Source: CAD feature listing. Evaluate the final solid. Frame: model axes, mm. Give positions to 0.01 mm unless a question says otherwise; leave off trailing zeros. Loops run counter-clockwise (first coordinate to the right, second up) from the corner with the lowest first, then second, coordinate; pieces in that order, holes last.
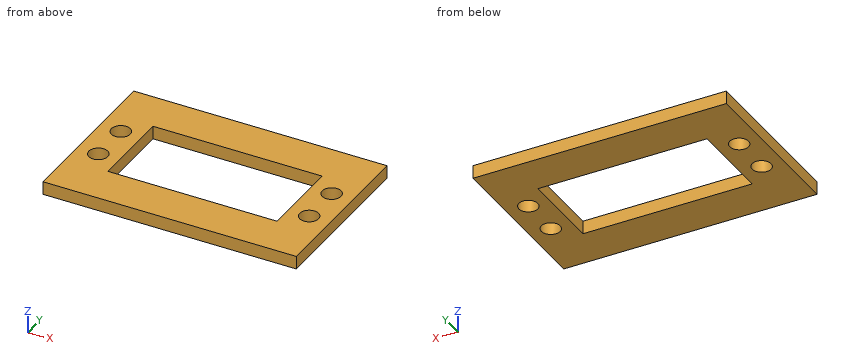
```python
from build123d import *

# Parameters (mm, degrees)
SKETCH1_W           = 61.214
SKETCH1_H           = 40.386
SKETCH1_W_2         = 40.894
SKETCH1_H_2         = 20.066
BOSS_EXTRUDE1_DEPTH = 3.175
SKETCH2_R           = 2.286
CUT_EXTRUDE1_DEPTH  = 4.175


with BuildPart() as part:
    # Sketch1 → Boss-Extrude1 (new body)
    with BuildSketch(Plane.XY):
        with Locations((20.447, 10.033)):
            Rectangle(SKETCH1_W, SKETCH1_H)
        with Locations((20.447, 10.033)):
            Rectangle(SKETCH1_W_2, SKETCH1_H_2, mode=Mode.SUBTRACT)
    extrude(amount=BOSS_EXTRUDE1_DEPTH)

    # Sketch2 → Cut-Extrude1 (cut, through all)
    with BuildSketch(Plane.XY.offset(3.175)):
        with Locations((-5.04, 15.033)):
            Circle(SKETCH2_R)
        with Locations((-5.04, 5.033)):
            Circle(SKETCH2_R)
        with Locations((45.934, 5.033)):
            Circle(SKETCH2_R)
        with Locations((45.934, 15.033)):
            Circle(SKETCH2_R)
    extrude(amount=-CUT_EXTRUDE1_DEPTH, mode=Mode.SUBTRACT)


solid = part.part
```
(1) Section A-A, the plane x = 38. Return the cut outline in (y, z) (3 decimals).
A:
outline: (-10.16, 0) - (0, 0) - (0, 3.175) - (-10.16, 3.175) - close; (20.066, 0) - (30.226, 0) - (30.226, 3.175) - (20.066, 3.175) - close
(2) Ray query, line 1 along Y through (x, z) = (46, 1.3); line 2 along Y through (x, z) = (33.5, 1.45); line 3 along X through (y, z) = (18, 0.5). Return the intervals inside material, ascending.
A:
line 1: y = -10.16 to 2.75, 7.32 to 12.75, 17.32 to 30.23
line 2: y = -10.16 to 0, 20.07 to 30.23
line 3: x = -10.16 to 0, 40.89 to 51.05
(3) Section B-B, the plane x = -6. Return the cut outline in (y, z) (3 decimals).
A:
outline: (-10.16, 0) - (2.958, 0) - (2.958, 3.175) - (-10.16, 3.175) - close; (7.108, 0) - (12.958, 0) - (12.958, 3.175) - (7.108, 3.175) - close; (17.108, 0) - (30.226, 0) - (30.226, 3.175) - (17.108, 3.175) - close
(4) Section D-D, the plane z = 0.95. Return the cut outline in (x, y).
A:
outline: (-10.16, -10.16) - (51.05, -10.16) - (51.05, 30.23) - (-10.16, 30.23) - close; hole circle Ø4.57 at (-5.04, 5.03); hole circle Ø4.57 at (-5.04, 15.03); hole (0, 0) - (40.89, 0) - (40.89, 20.07) - (0, 20.07) - close; hole circle Ø4.57 at (45.93, 5.03); hole circle Ø4.57 at (45.93, 15.03)
(5) Section C-C, the plane y = 14. Return the cut outline in (x, z) (3 decimals).
A:
outline: (-10.16, 0) - (-7.079, 0) - (-7.079, 3.175) - (-10.16, 3.175) - close; (-3.001, 0) - (0, 0) - (0, 3.175) - (-3.001, 3.175) - close; (40.894, 0) - (43.895, 0) - (43.895, 3.175) - (40.894, 3.175) - close; (47.973, 0) - (51.054, 0) - (51.054, 3.175) - (47.973, 3.175) - close
